Design review of the part shown in the three views and the two pictorial views. Dimensions are in mm from the part's minimum x, y and z. A direction names the side the tool comes from. Round coordinates to 2 decimals unless told otherwise and drop trailing zeros. Loops run counter-clockwise (first coordinate to the right, second up) from the corner with the lowest first, then second, coordinate; pieces in that order, holes last. Notation, with made-up numbers: M 81.25,-3 L 115.25,-3 A15 ccw 115.25,7 Z; hole C -30,45 d6. An arc over 180 degrees is marked long. One line per question, with ' | ' between items. Start each with the question number.
1) We need section D-D (z = 34.5). Give the boundary of the cut face in (x, y).
2) For pin 1 Ø10 at (x, z) = (19, 31.5) entering from -Y; pin 2 Ø1 at (y, z) = (20, 23) entering from +X, all flat-tipped, find the tip position at first contact; note any pin that passes through.
3) We need section C-C (y = 13). Give the boundary of the cut face in (x, z) (1 decimal), and give its area (3 significant figures).
4) We need section A-A (x = 13). Give the boundary of the cut face in (y, z).
5) For the marked faces 1 and 2, list the 3-axis set-ups (+Z, -Z, +X, -X, +Y, -Y) from which the entire face can be reached by the end or side of a thin tool; tool diameter is ignored.
6) For probe 1 along Z at (x, y) = (26.5, 26.5); probe 2 along X at (y, z) = (17.5, 26); probe 3 along Y at (x, z) = (28, 2.5) (1 decimal), list the stretches that pass through material, from the lowest coordinate up. Write a range as from..to.
7) Mouldability with a two-part tool opening along X and no side actions: class the marked faces 3, 4, 5 and 6 as pulls with the +X half, pulls with the -X half, needs draft (parallel to the pull), parting line crosses it, or undercut.
8) We need section B-B (x = 21.5). Give the boundary of the cut face in (y, z) (1 decimal).
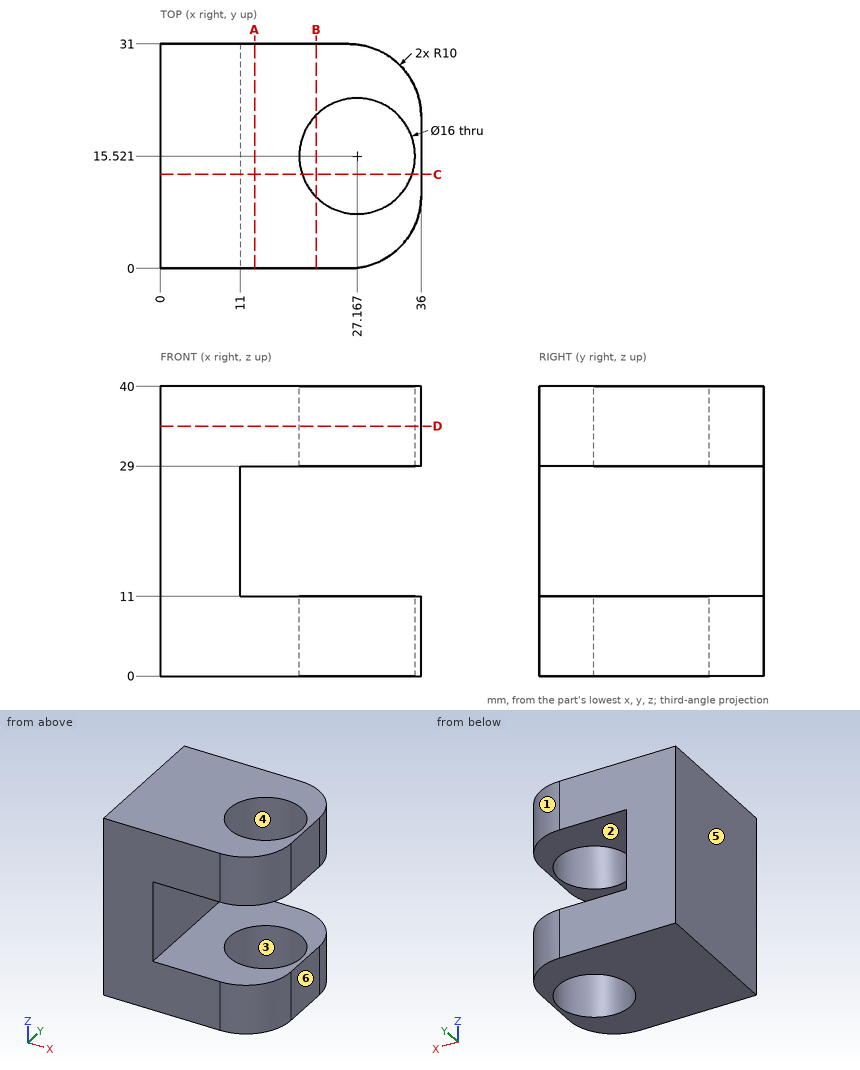
Answers below:
1) outline: M 0,0 L 26,0 A10 ccw 36,10 L 36,21 A10 ccw 26,31 L 0,31 Z; hole C 27.17,15.52 d16
2) pin 1: y = 0 | pin 2: x = 11
3) outline: M 0,0 L 19.6,0 L 19.6,11 L 11,11 L 11,29 L 19.6,29 L 19.6,40 L 0,40 Z; M 34.8,0 L 36,0 L 36,11 L 34.8,11 Z; M 34.8,29 L 36,29 L 36,40 L 34.8,40 Z | area: 656 mm^2
4) outline: M 0,0 L 31,0 L 31,11 L 0,11 Z; M 0,29 L 31,29 L 31,40 L 0,40 Z
5) face 1: +Z, -Z, +X, +Y | face 2: +X, +Y, -Y
6) probe 1: 0..11, 29..40 | probe 2: 0..11 | probe 3: 0.2..7.6, 23.5..30.8
7) face 3: undercut | face 4: undercut | face 5: pulls with the -X half | face 6: pulls with the +X half
8) outline: M 0,0 L 9.9,0 L 9.9,11 L 0,11 Z; M 0,29 L 9.9,29 L 9.9,40 L 0,40 Z; M 21.2,0 L 31,0 L 31,11 L 21.2,11 Z; M 21.2,29 L 31,29 L 31,40 L 21.2,40 Z
